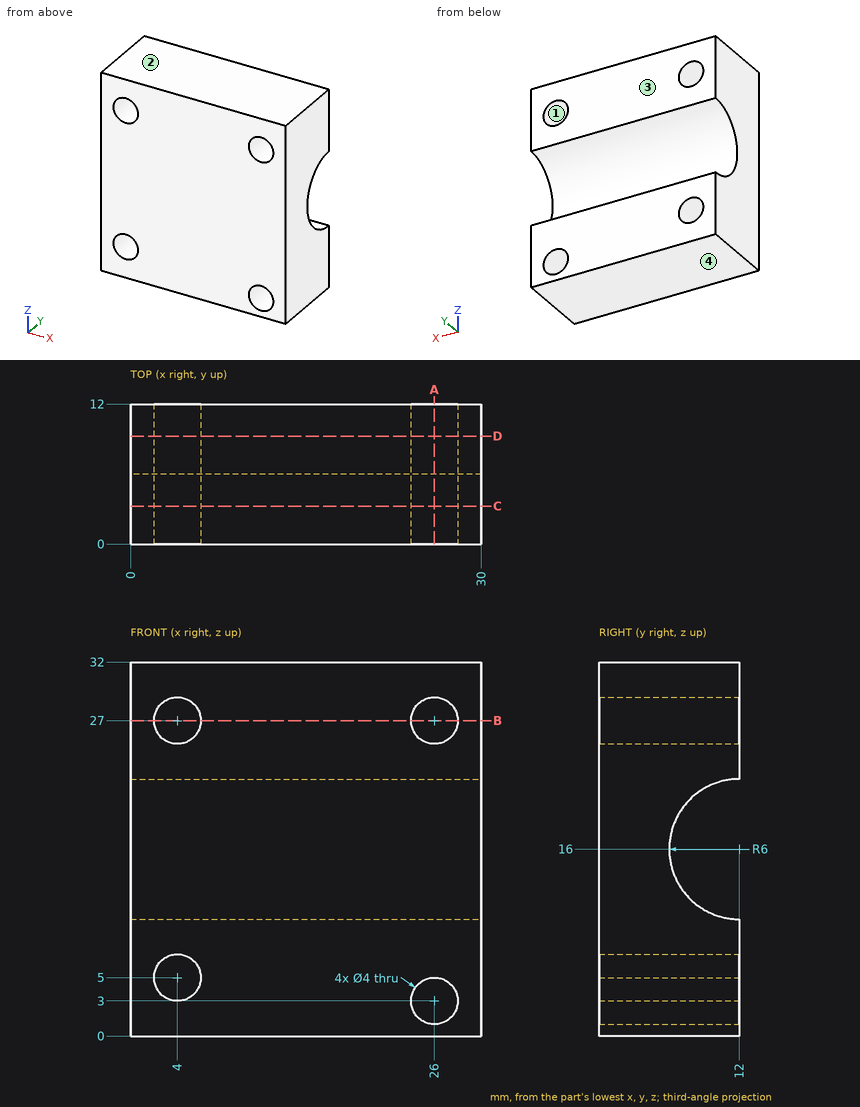
Design review of the part shown in the three views and the two pictorial views. Dimensions are in mm from the part's minimum x, y and z. Round coordinates to 2 decimals unless told otherwise and drop trailing zeros. Write each loop counter-clockwise with the first axis right and the second up, starting at its lowest first coordinate (ties: lowest second). Pieces come first, ordered by that corner, then holes. Notation, with made-up numbers: (79.25, -34.5) - (105.25, -34.5) arc R23 cw to (105.25, -23.5) - close; hole circle Ø10 at (72, 2). An arc over 180 degrees is marked (long way). Return JSON: item names as keys, results as strings. Group by question number.
Item 1: We need section B-B on z = 27. Write out the cut boundary in (x, y), and give its area (3 significant figures).
Item 2: We need section D-D on y = 9.25. Write out the cut boundary in (x, z).
Item 3: The part is to be moulded in two halves that separate along Z. For the marked faces 1, 2, 3 and 4, say which applies: pulls with the +Z half, pulls with the -Z half, needs draft (parallel to the pull), parting line crosses it, or undercut.
Item 4: Insertion check: P1, Ø3, axis at x = 4, z = 5, coming from the -Y side; P2, Ø10, axis at x = 20, z = 15.5, coming from the +Y side; P3, Ø6.5, axis at x = 26, z = 27, coming from the +Y side; P4, Ø4, axis at x = 22, z = 18, coming from the +Y side. Each pin has a flat end and moves straight along its axis. Give the tip position at first contact, or say it passes through.
Item 5: We need section C-C on y = 3.25. Write out the cut boundary in (x, z).
Item 6: For probe 1 along X at (y, z) = (7.25, 27); probe 2 along Z at (x, y) = (4, 5.5); probe 3 along Z at (x, y) = (27.75, 9), list the stretches that pass through material, from the lowest coordinate up. Write a range as [from, to].
Item 7: We need section A-A on x = 26. Write out the cut boundary in (y, z), and give its area (3 significant figures).
Model answer:
{
 "1": {"outline": "(0, 0) - (2, 0) - (2, 12) - (0, 12) - close; (6, 0) - (24, 0) - (24, 12) - (6, 12) - close; (28, 0) - (30, 0) - (30, 12) - (28, 12) - close", "area": "264 mm²"},
 "2": {"outline": "(0, 0) - (30, 0) - (30, 10.67) - (0, 10.67) - close; (0, 21.33) - (30, 21.33) - (30, 32) - (0, 32) - close; hole circle Ø4 at (4, 5); hole circle Ø4 at (4, 27); hole circle Ø4 at (26, 3); hole circle Ø4 at (26, 27)"},
 "3": {"face 1": "undercut", "face 2": "pulls with the +Z half", "face 3": "needs draft", "face 4": "pulls with the -Z half"},
 "4": {"P1": "passes through", "P2": "stops at y = 9.6", "P3": "stops at y = 12", "P4": "stops at y = 7.53"},
 "5": {"outline": "(0, 0) - (30, 0) - (30, 32) - (0, 32) - close; hole circle Ø4 at (4, 5); hole circle Ø4 at (4, 27); hole circle Ø4 at (26, 3); hole circle Ø4 at (26, 27)"},
 "6": {"probe 1": "x = [0, 2], [6, 24], [28, 30]", "probe 2": "z = [0, 3], [7, 25], [29, 32]", "probe 3": "z = [0, 2.03], [3.97, 10.8], [21.2, 26.03], [27.97, 32]"},
 "7": {"outline": "(0, 0) - (12, 0) - (12, 1) - (0, 1) - close; (0, 5) - (12, 5) - (12, 10) arc R6 cw to (12, 22) - (12, 25) - (0, 25) - close; (0, 29) - (12, 29) - (12, 32) - (0, 32) - close", "area": "231 mm²"}
}
